Could you check a few things on this drawing? It's one solid part, dimensions in mm from its lowest x, y, z. Round coordinates to 2 decimals unless told otherwise and drop trailing zeros. Write each loop counter-clockwise with the first axis right and the second up, starting at its lowest first coordinate (ties: lowest second). Pieces come first, ordered by that corner, then holes. Notation, with made-up numbers: (-23.5, 80) -> (31.5, 80) arc R24 ccw to (31.5, 104) -> close; hole circle Ø4 at (70, 52). An arc over 180 degrees is marked (long way). Answer as CSV lines item,"result".
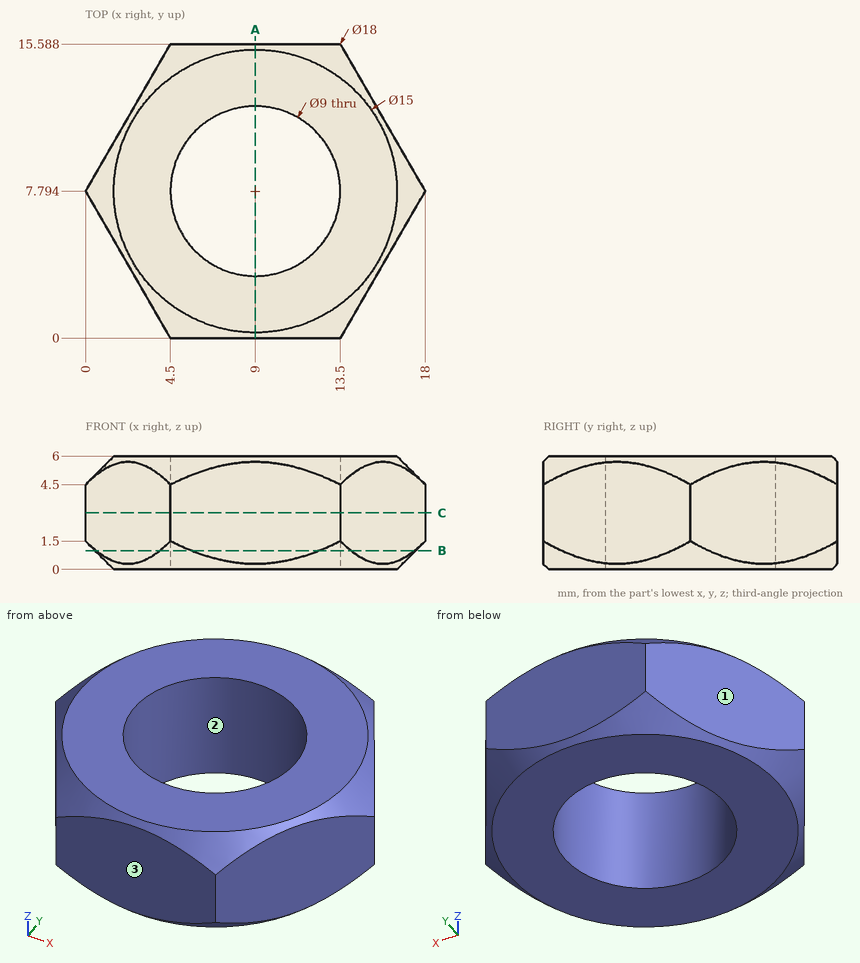
1. If we mould it in two halves opening along X, with no side actions, what happens to the marked faces 1, 2 and 3? For each: released by +X, released by -X, zero draft, split by the parting line, or undercut.
Numbers:
face 1,"released by -X"
face 2,"undercut"
face 3,"zero draft"
2. Suppose I cut it at B-B on z = 1. Please give me the cut outline in (x, y) (1 decimal).
Numbers:
outline,"(0.6, 6.8) -> (3.9, 1) arc R8.5 ccw to (5.6, 0) -> (12.4, 0) arc R8.5 ccw to (14.1, 1) -> (17.4, 6.8) arc R8.5 ccw to (17.4, 8.8) -> (14.1, 14.6) arc R8.5 ccw to (12.4, 15.6) -> (5.6, 15.6) arc R8.5 ccw to (3.9, 14.6) -> (0.6, 8.8) arc R8.5 ccw to start; hole circle Ø9 at (9, 7.8)"
3. If I drill on line 1 (Y direction, x = 9, z = 2.55) (1 decimal); line 2 (Y direction, x = 9.75, z = 4.75); line 3 (X direction, y = 10.75, z = 2.25) (1 decimal), over which ranges is the centre line in solid material (lowest first)?
Numbers:
line 1,"y = 0 to 3.3, 12.3 to 15.6"
line 2,"y = 0 to 3.36, 12.23 to 15.59"
line 3,"x = 1.7 to 5.6, 12.4 to 16.3"
4. Suppose I cut it at A-A on x = 9. Please give me the cut outline in (y, z) (1 decimal).
Numbers:
outline,"(0, 0.3) -> (0.3, 0) -> (3.3, 0) -> (3.3, 6) -> (0.3, 6) -> (0, 5.7) -> close; (12.3, 0) -> (15.3, 0) -> (15.6, 0.3) -> (15.6, 5.7) -> (15.3, 6) -> (12.3, 6) -> close"
5. For pin 1 Ø8 at (x, y) = (9, 7.79) entering from -Z; pin 2 Ø1.5 at (x, z) = (3, 2.5) entering from -Y, each with a flat end and sliding along its axis, tell me the tip position at first contact or that it passes through.
Numbers:
pin 1,"passes through"
pin 2,"stops at y = 1.3"
6. Suppose I cut it at C-C on z = 3. Please give me the cut outline in (x, y) (1 decimal), and give its area (3 significant figures).
Numbers:
outline,"(0, 7.8) -> (4.5, 0) -> (13.5, 0) -> (18, 7.8) -> (13.5, 15.6) -> (4.5, 15.6) -> close; hole circle Ø9 at (9, 7.8)"
area,"147 mm^2"
